The figure shows three views and two pictorial views of one solid part (mm, origin at its lowest corner). Answer the questions. A direction names the side the tool comes from. Coordinates: 2 decimals unless noted, no trailing zeros. Write each loop counter-clockwise with the first axis right and the second up, starting at its lowest first coordinate (ties: lowest second). Pieces come first, ordered by that corner, then holes. Notation, with made-up numbers: (-35.5, -12.5) - (-12.5, -12.5) arc R27 cw to (-12.5, 7.5) - close; hole circle Ø10 at (-9.5, 25). An arc over 180 degrees is marked (long way). Use a Markdown table: item, result. Add a question column.
(1) For a pull along X with two mould halves and no side action, classify the marked faces 1, 2 and 3 as released by +X, released by -X, zero draft, split by the parting line, or undercut.
(2) A tool of negligible diameter and unlimited length cuts with its end or side. For the marked faces 4, 5 and 6, from which of +Z, -Z, +X, -X, +Y, -Y can it reach the whole face along a straight path? Write none if from no direction.
(3) The part is cut by section B-B, the plane y = 20.5. Give the vertices of the cut face in (x, z) (1 decimal).
(4) Given pin 1 Ø2 at (y, z) = (18.5, 2) entering from +X; pin 2 Ø5 at (x, z) = (41.7, 6.27) entering from +Y; pin 3 Ø7 at (x, y) = (65.5, 15.5) entering from -Z; pin 4 Ø11.5 at (x, y) = (26, 9) entering from +Z, each flat-ended and moving along its own axis, determine where each tip first touches the part or whether it passes through.
(5) The part is cut by section A-A, the plane z = 7. Give the vertices of the cut face in (x, y), then the cut area to 3 significant figures.
(6) Find the intervals of material crossed by line 1 (X direction, y = 10.5, z = 6) (1 decimal); line 2 (Z direction, x = 22, y = 17.25); line 3 (X direction, y = 9, z = 8.5) (1 decimal), in increasing order. Write a range as from..to.
(7) The part is cut by section C-C, the plane x = 52. Give the vertices of the cut face in (y, z).
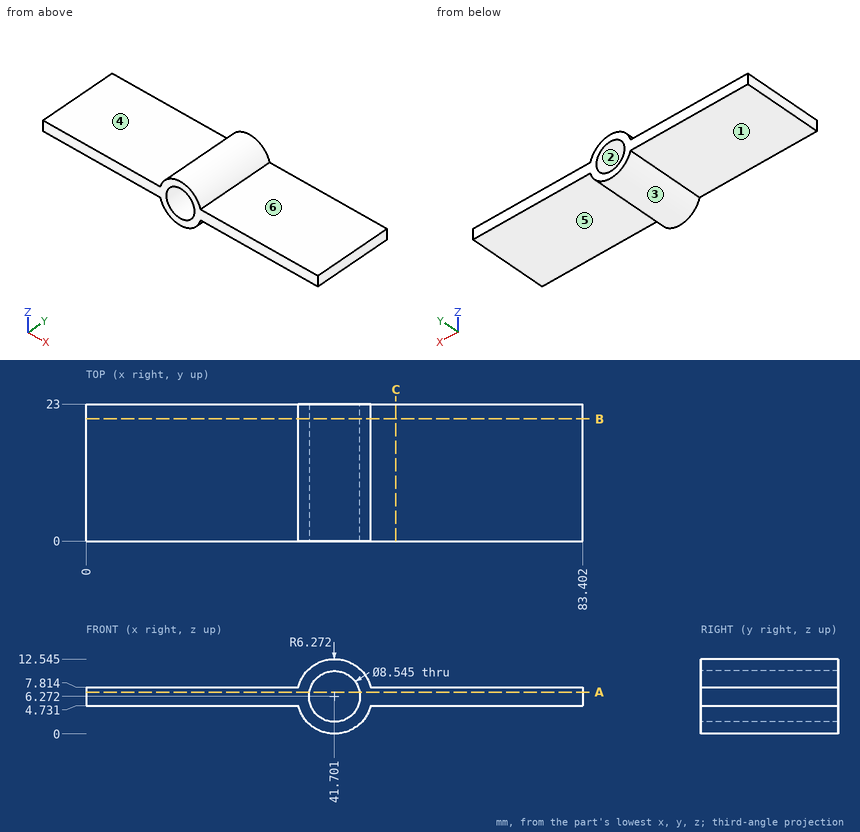
Model answer:
| question | item | result |
|---|---|---|
| 1 | face 1 | zero draft |
| 1 | face 2 | undercut |
| 1 | face 3 | split by the parting line |
| 2 | face 4 | +Z, -X, +Y, -Y |
| 2 | face 5 | -Z, +X, +Y, -Y |
| 2 | face 6 | +Z, +X, +Y, -Y |
| 3 | outline | (0, 4.7) - (35.6, 4.7) arc R6.3 ccw to (47.8, 4.7) - (83.4, 4.7) - (83.4, 7.8) - (47.8, 7.8) arc R6.3 ccw to (35.6, 7.8) - (0, 7.8) - close; hole circle Ø8.5 at (41.7, 6.3) |
| 4 | pin 1 | x = 47.05 |
| 4 | pin 2 | through |
| 4 | pin 3 | z = 4.73 |
| 4 | pin 4 | z = 7.81 |
| 5 | outline | (0, 0) - (37.49, 0) - (37.49, 23) - (0, 23) - close; (45.91, 0) - (83.4, 0) - (83.4, 23) - (45.91, 23) - close |
| 5 | area | 1,720 mm^2 |
| 6 | line 1 | 0..37.4, 46..83.4 |
| 6 | line 2 | 4.73..7.81 |
| 6 | line 3 | 35.8..38.1, 45.3..47.6 |
| 7 | outline | (0, 4.73) - (23, 4.73) - (23, 7.81) - (0, 7.81) - close |
